```python
from build123d import *

# Parameters (mm, degrees)
SKETCH_1_R          = 1.8
SKETCH_1_R_2        = 11.5
SKETCH_1_R_3        = 2.7
SKETCH_1_W          = 20.5
SKETCH_1_H          = 20.5
EXTRUDE_1_DEPTH     = 4
EXTRUDE_START       = 4
SKETCH_1_4_W        = 32
SKETCH_1_4_H        = 30
SKETCH_1_4_W_2      = 20.5
SKETCH_1_4_H_2      = 20.5
SKETCH_1_4_R        = 1.6
EXTRUDE_3_DEPTH     = 19.6
CUT_EXTRUDE_4_REACH = 103.737
SKETCH_8_R          = 2.4
SKETCH_9_R          = 5
SKETCH_9_R_2        = 2.7
EXTRUDE_4_DEPTH     = 7.7


with BuildPart() as part:
    # 草图1 → 凸台-拉伸1 (new body)
    with BuildSketch(Plane.XY):
        with BuildLine():
            ThreePointArc((-36, -25.5), (-31.606601718, -36.106601718), (-21, -40.5))
            Line((-21, -40.5), (21, -40.5))
            ThreePointArc((21, -40.5), (31.606601718, -36.106601718), (36, -25.5))
            Line((36, -25.5), (36, -14.034980384))
            ThreePointArc((36, -14.034980384), (38.3, -8.3), (36, -2.565019616))
            Line((36, -2.565019616), (36, 31.75))
            ThreePointArc((36, 31.75), (30.435028843, 45.185028843), (17, 50.75))
            Line((17, 50.75), (-17, 50.75))
            ThreePointArc((-17, 50.75), (-30.435028843, 45.185028843), (-36, 31.75))
            Line((-36, 31.75), (-36, -2.565019616))
            ThreePointArc((-36, -2.565019616), (-38.3, -8.3), (-36, -14.034980384))
            Line((-36, -14.034980384), (-36, -25.5))
        make_face()
        with Locations((15.5, -35)):
            Circle(SKETCH_1_R, mode=Mode.SUBTRACT)
        with Locations((0, -19.5)):
            Circle(SKETCH_1_R_2, mode=Mode.SUBTRACT)
        with Locations((15.5, -4)):
            Circle(SKETCH_1_R, mode=Mode.SUBTRACT)
        with Locations((-15.5, -35)):
            Circle(SKETCH_1_R, mode=Mode.SUBTRACT)
        with Locations((-15.5, -4)):
            Circle(SKETCH_1_R, mode=Mode.SUBTRACT)
        with Locations((-30, -8.3)):
            Circle(SKETCH_1_R_3, mode=Mode.SUBTRACT)
        with Locations((30, -8.3)):
            Circle(SKETCH_1_R_3, mode=Mode.SUBTRACT)
        with Locations((-29, 28.1)):
            Circle(SKETCH_1_R_3, mode=Mode.SUBTRACT)
        with Locations((29, 28.1)):
            Circle(SKETCH_1_R_3, mode=Mode.SUBTRACT)
        with Locations((0, 35.75)):
            Rectangle(SKETCH_1_W, SKETCH_1_H, mode=Mode.SUBTRACT)
    extrude(amount=EXTRUDE_1_DEPTH)

    # 草图1<4> → 凸台-拉伸3 (add)
    # profile 1 of 3: a face of its own
    with BuildSketch(Plane.XY.offset(EXTRUDE_START)):
        with Locations((0, 35.75)):
            Rectangle(SKETCH_1_4_W, SKETCH_1_4_H)
        with Locations((0, 35.75)):
            Rectangle(SKETCH_1_4_W_2, SKETCH_1_4_H_2, mode=Mode.SUBTRACT)
    # profile 2 of 3: a face of its own
    with BuildSketch(Plane.XY.offset(EXTRUDE_START)):
        with Locations((-13.2, 35.75)):
            Circle(SKETCH_1_4_R)
    # profile 3 of 3: a face of its own
    with BuildSketch(Plane.XY.offset(EXTRUDE_START)):
        with Locations((13.2, 35.75)):
            Circle(SKETCH_1_4_R)
    extrude(amount=EXTRUDE_3_DEPTH)

    # 草图8 → 切除-拉伸4 (cut, up to next)
    with BuildSketch(Plane(origin=(0, 50.75, 0), x_dir=(1, 0, 0), z_dir=(0, 1, 0)), mode=Mode.PRIVATE) as cut_extrude_4_sk1:
        with Locations(Location((0, -14, 0), (0, 0, 270))):
            Circle(SKETCH_8_R)
    cut_extrude_4_tool1 = extrude(cut_extrude_4_sk1.sketch, amount=-CUT_EXTRUDE_4_REACH, mode=Mode.PRIVATE) & part.part
    add(cut_extrude_4_tool1.solids().sort_by_distance((0, 50.75, 14))[0], mode=Mode.SUBTRACT)

    # 草图9 → 凸台-拉伸4 (add)
    # profile 1 of 4: a face of its own
    with BuildSketch(Plane.XY.offset(4)):
        with Locations(Location((-29, 28.1, 0), (0, 0, 180))):
            Circle(SKETCH_9_R)
        with Locations((-29, 28.1)):
            Circle(SKETCH_9_R_2, mode=Mode.SUBTRACT)
    # profile 2 of 4: a face of its own
    with BuildSketch(Plane.XY.offset(4)):
        with Locations(Location((-30, -8.3, 0), (0, 0, 180))):
            Circle(SKETCH_9_R)
        with Locations((-30, -8.3)):
            Circle(SKETCH_9_R_2, mode=Mode.SUBTRACT)
    # profile 3 of 4: a face of its own
    with BuildSketch(Plane.XY.offset(4)):
        with Locations(Location((30, -8.3, 0), (0, 0, 180))):
            Circle(SKETCH_9_R)
        with Locations(Location((30, -8.3, 0), (0, 0, 180))):
            Circle(SKETCH_9_R_2, mode=Mode.SUBTRACT)
    # profile 4 of 4: a face of its own
    with BuildSketch(Plane.XY.offset(4)):
        with Locations(Location((29, 28.1, 0), (0, 0, 180))):
            Circle(SKETCH_9_R)
        with Locations(Location((29, 28.1, 0), (0, 0, 180))):
            Circle(SKETCH_9_R_2, mode=Mode.SUBTRACT)
    extrude(amount=EXTRUDE_4_DEPTH)


solid = part.part
```
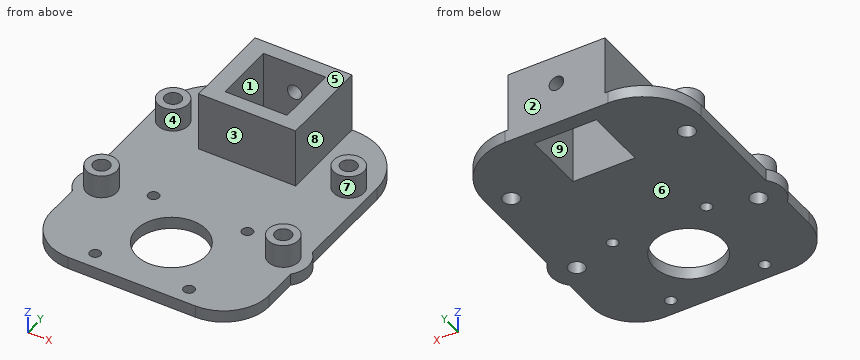
CAD build for the part. Positions are in the model's coordinates, mm. Face numbers are marked on the shaded views. A direction names the side the tool comes from. Round coordinates to 2 decimals unless told otherwise and drop trailing zeros. Loops run counter-clockwise (first coordinate to the right, second up) from the corner with the lowest first, then second, coordinate; pieces in that order, holes last. Notation, with made-up numbers: M -10,4 L 3,4 A16 ccw 3,8 Z; hole C 34,39 d9. An arc over 180 degrees is marked long. Use a Markdown table: item, result. Add a question column.
(1) Drill centre lines: line 1 (Y direction, x = 15.5, z = 3.05); line 2 (Y direction, x = 8.5, z = 22); line 3 (Y direction, x = 29, z = 6). Where is each one in solid material? Low to high.
(2) Cut at B-B (x = 0). Give the cut face in (y, z).
(3) Cut at A-A (z = 9). State how many separate pieces and enclosed holes the cut face has, and give its area (3 significant figures).
(4) Cut at C-C (y = 37.5). Give the cut face in (x, z).
(5) Which spindle directions (+Z, -Z, +X, -X, +Y, -Y) get a long thin tool onto all of the face, cutting with end or side? Do the marked faces 5, 6, 7, 8 and 9. Say none if no direction does.
(6) Cut at D-D (x = 30). Give the cut face in (y, z), and give its area (3 significant figures).
(7) Pull direction Y, two halves, no side cores. Call the marked faces 1, 2, 3 and 4: +Y half, -Y half, draft (parallel to the pull), parting line (faces both ways), or undercut.
(8) Flat gauge pins, fed straight in: pin 1 (4 mm diameter, centred on x = -15.5, y = -4, fed in from -Z); pin 2 (2 mm diameter, centred on y = 22, z = 3, fed in from -X); pin 3 (2 mm diameter, centred on y = -1, z = 7, fed in from -X); pin 4 (6 mm diameter, centred on y = 32, z = 13, fed in from -X). Where does each tip first touch, or does it go through?
Geometry says:
| question | item | result |
|---|---|---|
| 1 | line 1 | y = -40.5 to -36.8, -33.2 to -5.8, -2.2 to 50.75 |
| 1 | line 2 | y = 20.75 to 25.5, 46 to 50.75 |
| 1 | line 3 | y = -13.2 to -10.81, -5.79 to -3.4, 23.1 to 25.4, 30.8 to 33.1 |
| 2 | outline | M -40.5,0 L -31,0 L -31,4 L -40.5,4 Z; M -8,0 L 25.5,0 L 25.5,23.6 L 20.75,23.6 L 20.75,4 L -8,4 Z; M 46,0 L 50.75,0 L 50.75,11.6 L 46,11.6 Z; M 46,16.4 L 50.75,16.4 L 50.75,23.6 L 46,23.6 Z |
| 3 | separate pieces | 5 |
| 3 | enclosed holes | 5 |
| 3 | area | 762 mm² |
| 4 | outline | M -35.11,0 L -10.25,0 L -10.25,23.6 L -16,23.6 L -16,4 L -35.11,4 Z; M 10.25,0 L 35.11,0 L 35.11,4 L 16,4 L 16,23.6 L 10.25,23.6 Z |
| 5 | face 5 | +Z, +X, -X, +Y, -Y |
| 5 | face 6 | -Z, +X, -X, +Y, -Y |
| 5 | face 7 | +Z |
| 5 | face 8 | +Z, +Y, -Y |
| 5 | face 9 | +Z, -Z |
| 6 | outline | M -37.5,0 L -11,0 L -11,11.7 L -13.3,11.7 L -13.3,4 L -37.5,4 Z; M -5.6,0 L 25.59,0 L 25.59,11.7 L 23.2,11.7 L 23.2,4 L -3.3,4 L -3.3,11.7 L -5.6,11.7 Z; M 30.61,0 L 45.61,0 L 45.61,4 L 33,4 L 33,11.7 L 30.61,11.7 Z |
| 6 | area | 363 mm² |
| 7 | face 1 | undercut |
| 7 | face 2 | +Y half |
| 7 | face 3 | -Y half |
| 7 | face 4 | undercut |
| 8 | pin 1 | stops at z = 0 |
| 8 | pin 2 | stops at x = -36 |
| 8 | pin 3 | passes through |
| 8 | pin 4 | stops at x = -33.85 |
